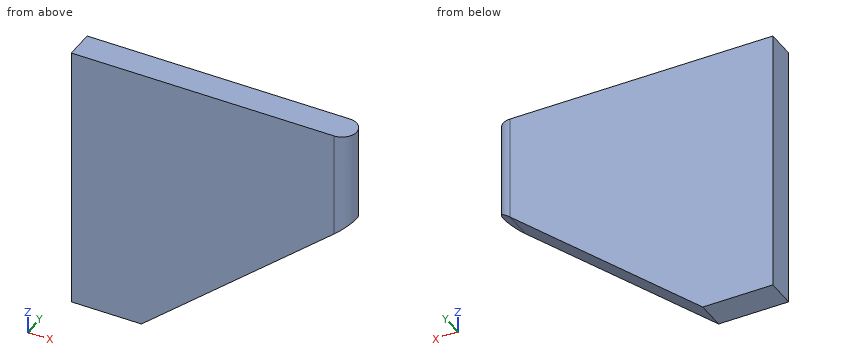
```python
from build123d import *

# Parameters (mm, degrees)
F1_DEPTH = 230
F3_DEPTH = 25.001


with BuildPart() as f1:
    # F0 (on Top) → F1 (new body)
    with BuildSketch(Plane.XY):
        with BuildLine():
            Line((0, 25), (0, 0))
            Line((0, 0), (225, 0))
            ThreePointArc((225, 0), (237.5, 12.5), (225, 25))
            Line((225, 25), (0, 25))
        make_face()
    extrude(amount=F1_DEPTH)

    # F2 (on face) → F3 (cut, through all)
    with BuildSketch(Plane.XZ):
        Polygon((237.5, 0), (237.5, 150), (225, 139.43662), (225, 0), align=None)
        Polygon((225, 0), (225, 139.43662), (60, 0), align=None)
    extrude(amount=-F3_DEPTH, mode=Mode.SUBTRACT)


solid = f1.part
```
The listing builds one solid part. Answer for the finished solid, in the listing's coordinates (mm). Give positions to 0.01 mm unless a question says otherwise; leave off trailing zeros. Order: outer loops, then holes, each group sorted by start corner. A loop starts at its lowest first (then second) coordinate and runs counter-clockwise, first axis right, second up.
Item 1: Given pin 1 Ø3 at (y, z) = (11.5, 31) entering from +X; pin 2 Ø1 at (y, z) = (17.5, 53.5) entering from +X, each flat-ended and moving along its own axis, determine where each tip first touches the part or whether it passes through.
From the geometry:
pin 1: stops at x = 98.46
pin 2: stops at x = 123.9
Item 2: The part is cut by section A-A, the plane z = 135. Give the vertices of the cut face in (x, y), and give its area (3 significant figures).
From the geometry:
outline: (0, 0) - (219.75, 0) - (219.75, 25) - (0, 25) - close
area: 5,490 mm2
Item 3: Find the intervals of material crossed by probe 1 along X at (y, z) = (14.5, 42.5); probe 2 along Z at (x, y) = (177.5, 22); probe 3 along X at (y, z) = (2.25, 202), in increasing order.
From the geometry:
probe 1: x = 0 to 110.29
probe 2: z = 99.3 to 230
probe 3: x = 0 to 232.15
Item 4: The part is cut by section C-C, the plane x = 187. Give the vertices of the cut face in (y, z), and give its area (3 significant figures).
From the geometry:
outline: (0, 107.32) - (25, 107.32) - (25, 230) - (0, 230) - close
area: 3,070 mm2
Item 5: The part is cut by section B-B, the plane y = 12.5. Give the vertices of the cut face in (x, z), and give its area (3 significant figures).
From the geometry:
outline: (0, 0) - (60, 0) - (237.5, 150) - (237.5, 230) - (0, 230) - close
area: 41,300 mm2
